For this review, take the finished solid that the model builds, in its own axes (mm). A direction names the side the tool comes from. Give positions to 0.01 mm unless a question says otherwise; leave off trailing zeros. Write each loop counter-clockwise with the first axis right and the second up, starting at its lowest first coordinate (ties: lowest second). Pieces come first, ordered by that corner, then holes. Notation, with made-up numbers: M 6.25,9 L 48.25,9 A19 ccw 48.25,19 Z; hole C -35.5,-13 d10. An arc over 180 degrees is marked long. Write item = value, one per line.
```python
from build123d import *

# Parameters (mm, degrees)
F0_W      = 51.3
F0_H      = 60.8
F0_R      = 1.8
F0_W_2    = 48.792678
F0_H_2    = 44.301098
F1_DEPTH  = 7
F1_FACE_W = 60.8
F1_FACE_H = 7
F2_DEPTH  = 15
F3_R      = 2.6
F4_DEPTH  = 25


with BuildPart() as f1:
    # F0 (on Top) → F1 (new body)
    with BuildSketch(Plane.XY):
        with Locations((25.65, -30.4)):
            Rectangle(F0_W, F0_H)
        with Locations((5.8, -55)):
            Circle(F0_R, mode=Mode.SUBTRACT)
        with Locations((47.3, -55)):
            Circle(F0_R, mode=Mode.SUBTRACT)
        with Locations((24.478404, -29.314266)):
            Rectangle(F0_W_2, F0_H_2, mode=Mode.SUBTRACT)
        with Locations((5.8, -4)):
            Circle(F0_R, mode=Mode.SUBTRACT)
        with Locations((47.3, -4)):
            Circle(F0_R, mode=Mode.SUBTRACT)
    extrude(amount=F1_DEPTH)

    # F1_face (on face) → F2 (join)
    with BuildSketch(Plane(origin=(0, -30.4, 3.5), x_dir=(0, -1, 0), z_dir=(-1, 0, 0))):
        Rectangle(F1_FACE_W, F1_FACE_H)
    extrude(amount=F2_DEPTH)

    # F3 (on face) → F4 (cut)
    with BuildSketch(Plane.XY.offset(7)):
        with Locations((-9.274096, -10)):
            Circle(F3_R)
        with Locations((-9.274096, -50.8)):
            Circle(F3_R)
    extrude(amount=-F4_DEPTH, mode=Mode.SUBTRACT)


solid = f1.part
```
1. We need section B-B, the plane z = 2. Write out the cut boundary in (x, y), then the cut area to 3 significant figures.
Responses:
outline = M -15,-60.8 L 51.3,-60.8 L 51.3,0 L -15,0 Z; hole C -9.27,-50.8 d5.2; hole C -9.27,-10 d5.2; hole M 0.08,-51.46 L 48.87,-51.46 L 48.87,-7.16 L 0.08,-7.16 Z; hole C 5.8,-55 d3.6; hole C 5.8,-4 d3.6; hole C 47.3,-55 d3.6; hole C 47.3,-4 d3.6
area = 1,790 mm2
2. Machinability: for faces 5 (the face through (0.082, -30, 3)), 6 (the face through (51.3, -31, 3)), which of the approach directions +Z, -Z, +X, -X, +Y, -Y give a long, thin tool a straight path to every point of the face, cutting with its end or side? Answer none if there is none.
Responses:
face_5 = +Z, -Z
face_6 = +Z, -Z, +X, +Y, -Y
3. For line 1 along Y through (x, z) = (5.8, 3.5); line 2 along Y through (x, z) = (43, 1.25); line 3 along X through (y, z) = (-5, 2.75), list the stretches that pass through material, from the lowest coordinate up. Write a range as from..to.
Responses:
line_1 = -60.8..-56.8, -53.2..-51.46, -7.16..-5.8, -2.2..0
line_2 = -60.8..-51.46, -7.16..0
line_3 = -15..4.3, 7.3..45.8, 48.8..51.3
4. Insertion check: P1, Ø3, axis at x = -9.27, y = -50.8, coming from the -Z side. The pin has a flat end and moves straight along its axis. Give the tip position at first contact, or say it passes through.
Responses:
P1 = through
5. We need section A-A, the plane y = -30. Write out the cut boundary in (x, z), then the cut area to 3 significant figures.
Responses:
outline = M -15,0 L 0.08,0 L 0.08,7 L -15,7 Z; M 48.87,0 L 51.3,0 L 51.3,7 L 48.87,7 Z
area = 123 mm2
6. We need section C-C, the plane x = 17. Write out the cut boundary in (y, z).
Responses:
outline = M -60.8,0 L -51.46,0 L -51.46,7 L -60.8,7 Z; M -7.16,0 L 0,0 L 0,7 L -7.16,7 Z
7. We need section D-D, the plane y = -55. Write out the cut boundary in (x, z), then the cut area to 3 significant figures.
Responses:
outline = M -15,0 L 4,0 L 4,7 L -15,7 Z; M 7.6,0 L 45.5,0 L 45.5,7 L 7.6,7 Z; M 49.1,0 L 51.3,0 L 51.3,7 L 49.1,7 Z
area = 414 mm2
8. The part is to be moulded in two halves that separate along Y. For faces 1 (the face through (49.017, -3.459, 3.451)), 2 (the face through (19, 0, 3)), 3 (the face through (19, -60.8, 3)), 4 (the face through (-1, -33, 0)), say which applies: +Y half, -Y half, draft (parallel to the pull), parting line (faces both ways), or undercut.
Responses:
face_1 = undercut
face_2 = +Y half
face_3 = -Y half
face_4 = draft
